Input: part model. Units: mm. Frame: model coordinates. A direction names the side the tool comes from. Coordinates: 2 decimals unless noted, no trailing zeros. Loops run counter-clockwise (first coordinate to the right, second up) from the corner with the lowest first, then second, coordinate; pieces in that order, holes last.
Item 1: Section A-A on y = 12.5. Return loops of the section in (x, z).
Item 2: Contact query for flat-ended pins moving along their axis: P1, Ø8, axis at x = 3.5, y = 7, coming from the +Z side; P2, Ø3, axis at y = 10.5, z = 6, coming from the -X side; P3, Ø2, axis at x = 0, y = 9, coming from the -Z side; P4, Ø2, axis at y = 18.5, z = 2, coming from the -X side. Output: stop coordinate, or through.
Item 3: Reachability of faces 4 (the cylindrical face through (48.699, 6.643, 6.479)), 5 (the cylindrical face through (5.5, 12.57, 2.54)) from +Z, -Z, +X, -X, +Y, -Y: full face, straight path, thin tool, end or side. Return the list, or none.
Item 4: Section B-B on x = 7. Return loops of the section in (y, z).
Item 5: Pull-direction query (Y, two-part tool) for faces 1 (the flat face through (25, 0, 2)), 2 (the cylindrical face through (0, 21, 3)), 3 (the cylindrical face through (-12.497, 12.775, 2.465)); classes: released by +Y, released by -Y, zero draft, split by the parting line, or undercut.
Item 6: Ray query, line 1 along Y through (x, z) = (50, 5.6); line 2 along Y through (x, z) = (0, 1.3); line 3 along Y through (x, z) = (1, 2.75). Return the intervals inside material, ascending.
Item 7: Section D-D on x = 45. Return loops of the section in (y, z), and give its area (3 significant figures).
Item 8: Section C-C on z = 3. Return loops of the section in (x, y).
```python
from build123d import *

# Parameters (mm, degrees)
SKETCH1_R           = 12.5
SKETCH1_W           = 50
SKETCH1_H           = 25
BOSS_EXTRUDE2_DEPTH = 5
CUT_EXTRUDE3_REACH  = 69.5
SKETCH3_R           = 4
SKETCH3_R_2         = 2.5
SKETCH3_3_R         = 7.5
SKETCH3_3_R_2       = 6
BOSS_EXTRUDE3_DEPTH = 3
CUT_EXTRUDE4_REACH  = 69.5
SKETCH3_4_R         = 1.5


with BuildPart() as part:
    # Sketch1 → Boss-Extrude2 (new body)
    with BuildSketch(Plane.XY):
        with Locations((0, 12.5)):
            Circle(SKETCH1_R)
        with Locations((50, 12.5)):
            Circle(SKETCH1_R)
        with Locations((25, 12.5)):
            Rectangle(SKETCH1_W, SKETCH1_H)
    extrude(amount=BOSS_EXTRUDE2_DEPTH)

    # Sketch3 → Cut-Extrude3 (cut, up to next)
    with BuildSketch(Plane.XY.offset(5), mode=Mode.PRIVATE) as cut_extrude3_sk1:
        with Locations((0, 12.5)):
            Circle(SKETCH3_R)
    cut_extrude3_tool1 = extrude(cut_extrude3_sk1.sketch, amount=-CUT_EXTRUDE3_REACH, mode=Mode.PRIVATE) & part.part
    # Sketch3 → Cut-Extrude3 (cut, up to next)
    with BuildSketch(Plane.XY.offset(5), mode=Mode.PRIVATE) as cut_extrude3_sk2:
        with Locations((50, 12.5)):
            Circle(SKETCH3_R_2)
    cut_extrude3_tool2 = extrude(cut_extrude3_sk2.sketch, amount=-CUT_EXTRUDE3_REACH, mode=Mode.PRIVATE) & part.part
    add(cut_extrude3_tool1.solids().sort_by_distance((0, 12.5, 5))[0], mode=Mode.SUBTRACT)
    add(cut_extrude3_tool2.solids().sort_by_distance((50, 12.5, 5))[0], mode=Mode.SUBTRACT)

    # Sketch3_3 → Boss-Extrude3 (add)
    with BuildSketch(Plane.XY.offset(5)):
        with Locations((50, 12.5)):
            Circle(SKETCH3_3_R)
        with Locations((50, 12.5)):
            Circle(SKETCH3_3_R_2, mode=Mode.SUBTRACT)
    extrude(amount=BOSS_EXTRUDE3_DEPTH)

    # Sketch3_4 → Cut-Extrude4 (cut, up to next)
    with BuildSketch(Plane.XY.offset(5), mode=Mode.PRIVATE) as cut_extrude4_sk1:
        with Locations((0, 19.5)):
            Circle(SKETCH3_4_R)
    cut_extrude4_tool1 = extrude(cut_extrude4_sk1.sketch, amount=-CUT_EXTRUDE4_REACH, mode=Mode.PRIVATE) & part.part
    # Sketch3_4 → Cut-Extrude4 (cut, up to next)
    with BuildSketch(Plane.XY.offset(5), mode=Mode.PRIVATE) as cut_extrude4_sk2:
        with Locations((0, 5.5)):
            Circle(SKETCH3_4_R)
    cut_extrude4_tool2 = extrude(cut_extrude4_sk2.sketch, amount=-CUT_EXTRUDE4_REACH, mode=Mode.PRIVATE) & part.part
    # Sketch3_4 → Cut-Extrude4 (cut, up to next)
    with BuildSketch(Plane.XY.offset(5), mode=Mode.PRIVATE) as cut_extrude4_sk3:
        with Locations((-7, 12.5)):
            Circle(SKETCH3_4_R)
    cut_extrude4_tool3 = extrude(cut_extrude4_sk3.sketch, amount=-CUT_EXTRUDE4_REACH, mode=Mode.PRIVATE) & part.part
    # Sketch3_4 → Cut-Extrude4 (cut, up to next)
    with BuildSketch(Plane.XY.offset(5), mode=Mode.PRIVATE) as cut_extrude4_sk4:
        with Locations((7, 12.5)):
            Circle(SKETCH3_4_R)
    cut_extrude4_tool4 = extrude(cut_extrude4_sk4.sketch, amount=-CUT_EXTRUDE4_REACH, mode=Mode.PRIVATE) & part.part
    add(cut_extrude4_tool1.solids().sort_by_distance((0, 19.5, 5))[0], mode=Mode.SUBTRACT)
    add(cut_extrude4_tool2.solids().sort_by_distance((0, 5.5, 5))[0], mode=Mode.SUBTRACT)
    add(cut_extrude4_tool3.solids().sort_by_distance((-7, 12.5, 5))[0], mode=Mode.SUBTRACT)
    add(cut_extrude4_tool4.solids().sort_by_distance((7, 12.5, 5))[0], mode=Mode.SUBTRACT)


solid = part.part
```
Results found:
1. outline: (-12.5, 0) - (-8.5, 0) - (-8.5, 5) - (-12.5, 5) - close; (-5.5, 0) - (-4, 0) - (-4, 5) - (-5.5, 5) - close; (4, 0) - (5.5, 0) - (5.5, 5) - (4, 5) - close; (8.5, 0) - (47.5, 0) - (47.5, 5) - (44, 5) - (44, 8) - (42.5, 8) - (42.5, 5) - (8.5, 5) - close; (52.5, 0) - (62.5, 0) - (62.5, 5) - (57.5, 5) - (57.5, 8) - (56, 8) - (56, 5) - (52.5, 5) - close
2. P1: stops at z = 5
2. P2: stops at x = -12.47
2. P3: stops at z = 0
2. P4: stops at x = -11.46
3. face 4: +Z
3. face 5: +Z, -Z
4. outline: (0, 0) - (11, 0) - (11, 5) - (0, 5) - close; (14, 0) - (25, 0) - (25, 5) - (14, 5) - close
5. face 1: released by -Y
5. face 2: undercut
5. face 3: split by the parting line
6. line 1: y = 5 to 6.5, 18.5 to 20
6. line 2: y = 0 to 4, 7 to 8.5, 16.5 to 18, 21 to 25
6. line 3: y = 0 to 4.38, 6.62 to 8.63, 16.37 to 18.38, 20.62 to 25
7. outline: (0, 0) - (25, 0) - (25, 5) - (18.09, 5) - (18.09, 8) - (15.82, 8) - (15.82, 5) - (9.18, 5) - (9.18, 8) - (6.91, 8) - (6.91, 5) - (0, 5) - close
7. area: 139 mm2
8. outline: (0, 0) - (50, 0) arc R12.5 ccw to (50, 25) - (0, 25) arc R12.5 ccw to start; hole circle Ø3 at (-7, 12.5); hole circle Ø8 at (0, 12.5); hole circle Ø3 at (0, 5.5); hole circle Ø3 at (0, 19.5); hole circle Ø3 at (7, 12.5); hole circle Ø5 at (50, 12.5)
